from build123d import *

# Parameters (mm, degrees)
SKETCH1_R           = 3.175
BOSS_EXTRUDE2_DEPTH = 6.35


with BuildPart() as part:
    # Sketch1 → Boss-Extrude2 (new body)
    with BuildSketch(Plane(origin=(0, 0, 0), x_dir=(1, 0, 0), z_dir=(0, 1, 0))):
        with BuildLine():
            Line((-125.579322034, 0), (128.420677966, 0))
            ThreePointArc((128.420677966, 0), (137.400934087, 3.719743879), (141.120677966, 12.7))
            Line((141.120677966, 12.7), (141.120677966, 148.007538959))
            ThreePointArc((141.120677966, 148.007538959), (140.423079494, 152.158726448), (138.406920869, 155.853872669))
            Line((138.406920869, 155.853872669), (11.406920869, 317.490236305))
            ThreePointArc((11.406920869, 317.490236305), (1.420677966, 322.343902596), (-8.565564937, 317.490236305))
            Line((-8.565564937, 317.490236305), (-135.565564937, 155.853872669))
            ThreePointArc((-135.565564937, 155.853872669), (-137.581723562, 152.158726448), (-138.279322034, 148.007538959))
            Line((-138.279322034, 148.007538959), (-138.279322034, 12.7))
            ThreePointArc((-138.279322034, 12.7), (-134.559578155, 3.719743879), (-125.579322034, 0))
        make_face()
        with Locations(Location((1.420677966, 296.943902596, 0), (0, 0, 270))):
            Circle(SKETCH1_R, mode=Mode.SUBTRACT)
        with Locations(Location((-12.295062697, 277.893902596, 0), (0, 0, 270))):
            Circle(SKETCH1_R, mode=Mode.SUBTRACT)
        with Locations(Location((14.258408226, 277.893902596, 0), (0, 0, 270))):
            Circle(SKETCH1_R, mode=Mode.SUBTRACT)
        with Locations(Location((1.420677966, 258.843902596, 0), (0, 0, 270))):
            Circle(SKETCH1_R, mode=Mode.SUBTRACT)
        with Locations(Location((-125.579322034, 148.007538959, 0), (0, 0, 270))):
            Circle(SKETCH1_R, mode=Mode.SUBTRACT)
        with Locations(Location((128.420677966, 148.007538959, 0), (0, 0, 270))):
            Circle(SKETCH1_R, mode=Mode.SUBTRACT)
        with Locations(Location((128.420677966, 12.7, 0), (0, 0, 270))):
            Circle(SKETCH1_R, mode=Mode.SUBTRACT)
        with Locations(Location((-125.579322034, 12.7, 0), (0, 0, 270))):
            Circle(SKETCH1_R, mode=Mode.SUBTRACT)
    extrude(amount=BOSS_EXTRUDE2_DEPTH)


solid = part.part
The model under review builds one solid part; all positions refer to its coordinate system, in mm. Round coordinates to 2 decimals unless told otherwise and drop trailing zeros. Write each loop counter-clockwise with the first axis right and the second up, starting at its lowest first coordinate (ties: lowest second). Pieces come first, ordered by that corner, then holes. Notation, with made-up numbers: M -18.5,-36 L 5.5,-36 A30 cw 5.5,-1 Z; hole C 88.25,-20 d7. An arc over 180 degrees is marked long. Answer as CSV lines item,"result". Start each with the question number.
Q1. Consider section C-C, the plane x = 53. Give the boundary of the cut face in (y, z).
Q2. Consider section B-B, the plane x = 116. Give the boundary of the cut face in (y, z), then the cut area to 3 significant figures.
Q3. The part is to be moulded in two halves that separate along Y. For faces 1 (the face through (-71.18, 3.13, -237.8)), 2 (the face through (-1, 6.35, -128)), 3 (the face through (-1, 0, -128)), say which applies: +Y half, -Y half, draft (parallel to the pull), parting line (faces both ways), or undercut.
Q4. Consider section A-A, the plane y = 3.25. State how many separate pieces and enclosed holes the cut face has, then the cut area to 3 significant figures.
Q5. Clearance check with flat-ended pins moving along their axes: P1, Ø1.5, axis at y = 3.5, z = -254.5, coming from the +X side; P2, Ø2, axis at y = 2, z = -168.5, coming from the +X side; P3, Ø2, axis at x = 25.5, y = 5, coming from the -Z side. State where each tip first meets the part, or that it passes through.
Q6. Wall thickness on line 1 along X through (y, z) = (4, -278); line 2 along Z through (x, y) = (0, 1.25); line 3 along X through (y, z) = (1.5, -277): over which ranges is each line inside the solid? List them lowest first.
Result set:
1,outline,"M 0,-264.55 L 6.35,-264.55 L 6.35,0 L 0,0 Z"
2,outline,"M 0,-184.37 L 6.35,-184.37 L 6.35,0 L 0,0 Z"
2,area,"1,170 mm²"
3,face 1,"draft"
3,face 2,"+Y half"
3,face 3,"-Y half"
4,separate pieces,"1"
4,enclosed holes,"8"
4,area,"67,000 mm²"
5,P1,"stops at x = 61.49"
5,P2,"stops at x = 129.26"
5,P3,"stops at z = -300.83"
6,line 1,"x = -39.59 to -15.47, -9.12 to 11.09, 17.43 to 42.43"
6,line 2,"z = -322.26 to -299.78, -294.1 to -261.68, -256 to 0"
6,line 3,"x = -40.38 to -15.34, -9.25 to 11.21, 17.3 to 43.22"
